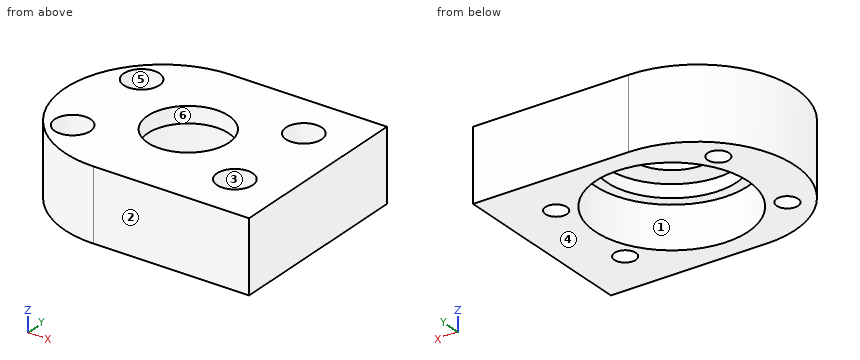
```python
from build123d import *

# Parameters (mm, degrees)
SKETCH_1_R                = 12.5
EXTRUDE_1_DEPTH           = 22
HOLE_WIZARD_1_D           = 6.6
HOLE_WIZARD_1_CBORE_D     = 11
HOLE_WIZARD_1_CBORE_DEPTH = 6.8
SKETCH_5_R                = 23.5
CUT_EXTRUDE_1_DEPTH       = 13
SKETCH_6_R                = 20
CUT_EXTRUDE_2_DEPTH       = 4


with BuildPart() as part:
    # 草图1 → 凸台-拉伸1 (new body)
    with BuildSketch(Plane.XY):
        with BuildLine():
            Line((-8, 30), (40, 30))
            Line((40, 30), (40, -30))
            Line((40, -30), (-8, -30))
            ThreePointArc((-8, -30), (-38, 0), (-8, 30))
        make_face()
        Circle(SKETCH_1_R, mode=Mode.SUBTRACT)
    extrude(amount=EXTRUDE_1_DEPTH)

    # 打孔尺寸(%根据)内六角圆柱头螺钉的类型1 (through all)
    with Locations(Plane(origin=(-25, 15, 22), x_dir=(1, 0, 0), z_dir=(0, 0, 1))):
        with Locations((0, 0), (0, -30), (50, 0), (50, -30)):
            CounterBoreHole(HOLE_WIZARD_1_D / 2, HOLE_WIZARD_1_CBORE_D / 2, HOLE_WIZARD_1_CBORE_DEPTH)

    # 草图5 → 切除-拉伸1 (cut)
    with BuildSketch(Plane(origin=(0, 0, 0), x_dir=(-1, 0, 0), z_dir=(0, 0, -1))):
        Circle(SKETCH_5_R)
    extrude(amount=-CUT_EXTRUDE_1_DEPTH, mode=Mode.SUBTRACT)

    # 草图6 → 切除-拉伸2 (cut)
    with BuildSketch(Plane(origin=(0, 0, 13), x_dir=(-1, 0, 0), z_dir=(0, 0, -1))):
        Circle(SKETCH_6_R)
    extrude(amount=-CUT_EXTRUDE_2_DEPTH, mode=Mode.SUBTRACT)


solid = part.part
```
Check sheet for the modelled part. Datum: model origin and axes. Units: mm. Face numbers are marked on the shaded views. A direction names the side the tool comes from. Round coordinates to 2 decimals unless told otherwise and drop trailing zeros. Loops run counter-clockwise (first coordinate to the right, second up) from the corner with the lowest first, then second, coordinate; pieces in that order, holes last. Notation, with made-up numbers: (65, -22) - (92, -22) arc R23 ccw to (92, 2) - close; hole circle Ø9 at (0.5, 12). An arc over 180 degrees is marked (long way). Answer as a JSON object with one key per item and string values. Group by question number.
Q1. Sectioned sample at D-D, the plane y = 0. Enter the section's corners in (x, z).
Q2. Sectioned sample at C-C, the plane z = 2. Enter the section's corners in (x, y), plus the area to 3 significant figures.
Q3. Scan lines: line 1 along X through (y, z) = (0, 20.4); line 2 along Y through (x, z) = (25.5, 13.25); line 3 along Y through (x, z) = (0, 20.75). Record each from-to range of solid material in increasing order. Write a range as [from, to].
Q4. Gauge pin test, flat ends, axial feed: P1, Ø5, axis at y = -2.5, z = 14.5, coming from the -X side; P2, Ø8, axis at x = 21.5, y = 23, coming from the -Z side; P3, Ø20, axis at x = 8, y = -4, coming from the -Z side; P4, Ø6.5, axis at x = 25, y = -15, coming from the +Z side. Record the tip position at first contact, or that the pin passes through.
Q5. Set-up check for the marked faces 5 and 6: record each of +Z, -Z, +X, -X, +Y, -Y from which the full face is reachable in a straight line by a thin tool's end or side.
Q6. Sectioned sample at B-B, the plane x = 0. Enter the section's corners in (y, z), plus the area to 3 significant figures.
Q7. Sectioned sample at A-A, the plane x = 25. Enter the section's corners in (y, z), plus the area to 3 significant figures.
Q8. Mould release check, pull along Y, two halves, no side actions. Record for the marked faces 1, 2, 3 and 4: released by +Y, released by -Y, zero draft, split by the parting line, or undercut.
Solution:
{
 "1": {"outline": "(-38, 0) - (-23.5, 0) - (-23.5, 13) - (-20, 13) - (-20, 17) - (-12.5, 17) - (-12.5, 22) - (-38, 22) - close; (12.5, 17) - (20, 17) - (20, 13) - (23.5, 13) - (23.5, 0) - (40, 0) - (40, 22) - (12.5, 22) - close"},
 "2": {"outline": "(-8, -30) - (40, -30) - (40, 30) - (-8, 30) arc R30 ccw to start; hole circle Ø6.6 at (-25, -15); hole circle Ø6.6 at (-25, 15); hole circle Ø47 at (0, 0); hole circle Ø6.6 at (25, -15); hole circle Ø6.6 at (25, 15)", "area": "2,420 mm²"},
 "3": {"line 1": "x = [-38, -12.5], [12.5, 40]", "line 2": "y = [-30, -18.26], [-11.74, 11.74], [18.26, 30]", "line 3": "y = [-30, -12.5], [12.5, 30]"},
 "4": {"P1": "stops at x = -38", "P2": "stops at z = 0", "P3": "stops at z = 17", "P4": "passes through"},
 "5": {"face 5": "+Z", "face 6": "+Z, -Z"},
 "6": {"outline": "(-30, 0) - (-23.5, 0) - (-23.5, 13) - (-20, 13) - (-20, 17) - (-12.5, 17) - (-12.5, 22) - (-30, 22) - close; (12.5, 17) - (20, 17) - (20, 13) - (23.5, 13) - (23.5, 0) - (30, 0) - (30, 22) - (12.5, 22) - close", "area": "424 mm²"},
 "7": {"outline": "(-30, 0) - (-18.3, 0) - (-18.3, 15.2) - (-20.5, 15.2) - (-20.5, 22) - (-30, 22) - close; (-11.7, 0) - (11.7, 0) - (11.7, 15.2) - (9.5, 15.2) - (9.5, 22) - (-9.5, 22) - (-9.5, 15.2) - (-11.7, 15.2) - close; (18.3, 0) - (30, 0) - (30, 22) - (20.5, 22) - (20.5, 15.2) - (18.3, 15.2) - close", "area": "970 mm²"},
 "8": {"face 1": "undercut", "face 2": "released by -Y", "face 3": "undercut", "face 4": "zero draft"}
}
